Verification items for the finished model (mm, model axes). Face numbers are marked on the shaded views. A direction names the side the tool comes from. Coordinates: 2 decimals unless noted, no trailing zeros. Order: outer loops, then holes, each group sorted by start corner. A loop starts at its lowest first (then second) coordinate and runs counter-clockwise, first axis right, second up. Notation, with made-up numbers: (-10.75, 83.25) - (-0.75, 83.25) arc R20 ccw to (-0.75, 92.25) - close; hole circle Ø10 at (24, 66). An arc over 180 degrees is marked (long way). Answer as CSV lines item,"result". Start each with the question number.
1. Section check D-D (z = -3). Record the cut outline in (x, y), and give its area (3 significant figures).
2. Section check B-B (z = 21.5). Record the cut outline in (x, y), and give its area (3 significant figures).
3. Section check C-C (x = 15). Record the cut outline in (y, z).
4. Set-up check for the marked faces 1, 2 and 3: record each of +Z, -Z, +X, -X, +Y, -Y from which the full face is reachable in a straight line by a thin tool's end or side.
5. Material ranges on L1, parallel to Y at x = -2.25, z = 41.45; L2, parallel to Y at x = 4.5, z = 42.55; L3, parallel to Z at x = -16, y = -5, recorded low to high. Write a range as [from, to].
6. Go/stop test with flat-tipped pins: pin 1 (1.9 mm diameter, centred on x = 14.5, y = 0, fed in from +Z); pin 2 (3.5 mm diameter, centred on x = 0.5, z = 28, fed in from +Y); pin 3 (0.9 mm diameter, centred on x = -0.39, y = 4.51, fed in from +Z); pin 4 (10.5 mm diameter, centred on x = 0.5, y = -1.5, fed in from +Z). Record where each tip stops, or that it passes through.
from build123d import *

# Parameters (mm, degrees)
SKETCH_1_R          = 17.5
EXTRUDE_1_DEPTH     = 27.2
SKETCH_2_R          = 15.8
EXTRUDE_2_DEPTH     = 11
SKETCH_3_W          = 22
SKETCH_3_H          = 22
EXTRUDE_3_DEPTH     = 3
SKETCH_4_R          = 10
EXTRUDE_4_DEPTH     = 12.7
SKETCH_5_R          = 1.2
CUT_EXTRUDE_1_DEPTH = 10
EXTRUDE_START       = -1.5
EXTRUDE_5_DEPTH     = 1.5
SKETCH_8_R          = 2.5
CUT_EXTRUDE_2_DEPTH = 1.8
SKETCH_9_R          = 0.75
CUT_EXTRUDE_3_DEPTH = 2


with BuildPart() as part:
    # 草图1 → 凸台-拉伸1 (new body)
    with BuildSketch(Plane.XY):
        Circle(SKETCH_1_R)
    extrude(amount=EXTRUDE_1_DEPTH)

    # 草图2 → 凸台-拉伸2 (add)
    with BuildSketch(Plane(origin=(0, 0, 0), x_dir=(-1, 0, 0), z_dir=(0, 0, -1))):
        with Locations(Location((0, 0, 0), (0, 0, 180))):
            Circle(SKETCH_2_R)
    extrude(amount=EXTRUDE_2_DEPTH)

    # 草图3 → 凸台-拉伸3 (add)
    with BuildSketch(Plane.XY.offset(27.2)):
        Rectangle(SKETCH_3_W, SKETCH_3_H)
    extrude(amount=EXTRUDE_3_DEPTH)

    # 草图4 → 凸台-拉伸4 (add)
    with BuildSketch(Plane.XY.offset(30.2)):
        with Locations(Location((0, 0, 0), (0, 0, 180))):
            Circle(SKETCH_4_R)
    extrude(amount=EXTRUDE_4_DEPTH)

    # 草图5 → 切除-拉伸1 (cut)
    with BuildSketch(Plane.XY.offset(27.2)):
        with Locations((0, -14.5)):
            Circle(SKETCH_5_R)
        with Locations((-14.5, 0)):
            Circle(SKETCH_5_R)
        with Locations((0, 14.5)):
            Circle(SKETCH_5_R)
        with Locations((14.5, 0)):
            Circle(SKETCH_5_R)
    extrude(amount=-CUT_EXTRUDE_1_DEPTH, mode=Mode.SUBTRACT)

    # 草图6 → 凸台-拉伸5 (add)
    with BuildSketch(Plane.XY.offset(18.2).offset(EXTRUDE_START)):
        with BuildLine():
            Line((-9, 15.00833102), (-9, 21.70833102))
            Line((-9, 21.70833102), (9, 21.70833102))
            Line((9, 21.70833102), (9, 15.00833102))
            ThreePointArc((9, 15.00833102), (0, 17.5), (-9, 15.00833102))
        make_face()
    extrude(amount=EXTRUDE_5_DEPTH)

    # 草图8 → 切除-拉伸2 (cut)
    with BuildSketch(Plane.XY.offset(42.9)):
        Circle(SKETCH_8_R)
    extrude(amount=-CUT_EXTRUDE_2_DEPTH, mode=Mode.SUBTRACT)

    # 草图9 → 切除-拉伸3 (cut)
    with BuildSketch(Plane.XY.offset(42.9)):
        with Locations((4.5, 0)):
            Circle(SKETCH_9_R)
        with Locations((4.106443914, -1.914866245)):
            Circle(SKETCH_9_R)
        with Locations((-2.25, -3.897114317)):
            Circle(SKETCH_9_R)
        with Locations((-3.71154477, -2.598851626)):
            Circle(SKETCH_9_R)
        with Locations((-2.25, 3.897114317)):
            Circle(SKETCH_9_R)
        with Locations((-0.394899144, 4.513717871)):
            Circle(SKETCH_9_R)
    extrude(amount=-CUT_EXTRUDE_3_DEPTH, mode=Mode.SUBTRACT)


solid = part.part
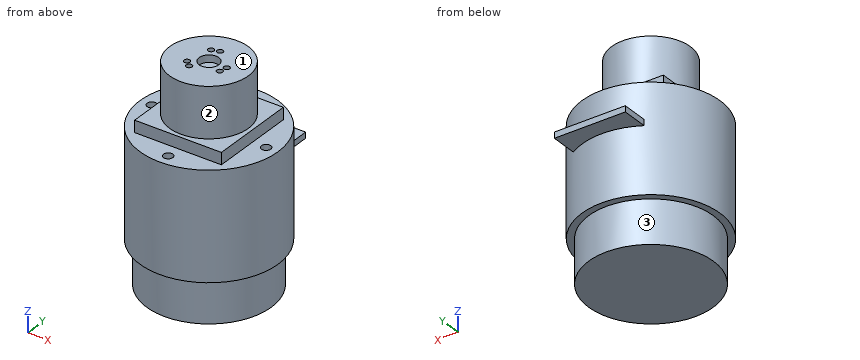
Evaluation:
1,outline,"circle Ø31.6 at (0, 0)"
1,area,"784 mm²"
2,outline,"circle Ø35 at (0, 0); hole circle Ø2.4 at (-14.5, 0); hole circle Ø2.4 at (0, -14.5); hole circle Ø2.4 at (0, 14.5); hole circle Ø2.4 at (14.5, 0)"
2,area,"944 mm²"
3,outline,"(-9.01, 0) - (-4.96, 0) - (-4.96, -11) - (4.96, -11) - (4.96, 0) - (9.01, 0) - (9.01, 27.2) - (1.09, 27.2) - (1.09, 17.2) - (-1.09, 17.2) - (-1.09, 27.2) - (-9.01, 27.2) - close"
4,face 1,"+Z, +X, -X, +Y, -Y"
4,face 2,"+Z"
4,face 3,"-Z"
5,L1,"y = [-9.74, -4.65], [-3.15, -1.09], [1.09, 3.15], [4.65, 9.74]"
5,L2,"y = [-8.93, -2.55], [-1.28, -0.75], [0.75, 8.93]"
5,L3,"z = [0, 27.2]"
6,pin 1,"stops at z = 17.2"
6,pin 2,"stops at y = 17.5"
6,pin 3,"stops at z = 40.9"
6,pin 4,"stops at z = 42.9"
